Verification items for the finished model (mm, model axes). A direction names the side the tool comes from. Round coordinates to 2 decimals unless told otherwise and drop trailing zeros. Write each loop counter-clockwise with the first axis right and the second up, starting at its lowest first coordinate (ties: lowest second). Pieces come first, ordered by that corner, then holes. Notation, with made-up numbers: (-20.75, 0.5) - (13.25, 0.5) arc R8 cw to (13.25, 15.5) - close; hole circle Ø7 at (-33.5, -7). An arc over 180 degrees is marked (long way). Answer as a JSON object with one key per item and string values.
```python
from build123d import *

# Parameters (mm, degrees)
SKETCH1_R                = 13.6525
SKETCH1_R_2              = 10.668
BOSS_EXTRUDE1_DEPTH      = 63.5
SKETCH3_R                = 10.668
CUT_EXTRUDE2_DEPTH       = 69.85
BOSS_EXTRUDE2_REACH      = 81.247
BOSS_EXTRUDE2_END_RADIUS = 13.6525
SKETCH4_R                = 13.6525
SKETCH4_R_2              = 10.668
SKETCH5_W                = 1.905
SKETCH5_H                = 1.27
SKETCH6_W                = 1.27
SKETCH6_H                = 1.905
SKETCH7_W                = 1.27
SKETCH7_H                = 1.905


with BuildPart() as part:
    # Sketch1 → Boss-Extrude1 (new body)
    with BuildSketch(Plane(origin=(0, 0, 0), x_dir=(1, 0, 0), z_dir=(0, 1, 0))):
        with Locations(Location((0, 0, 0), (0, 0, 270))):
            Circle(SKETCH1_R)
        with Locations(Location((0, 0, 0), (0, 0, 270))):
            Circle(SKETCH1_R_2, mode=Mode.SUBTRACT)
    extrude(amount=BOSS_EXTRUDE1_DEPTH)

    # Sketch3 → Cut-Extrude2 (cut)
    with BuildSketch(Plane.XY):
        with Locations((0, 31.75)):
            Circle(SKETCH3_R)
    extrude(amount=-CUT_EXTRUDE2_DEPTH, mode=Mode.SUBTRACT)

    # Boss-Extrude2: up to this cylinder (the profile starts outside it)
    boss_extrude2_end = Plane(origin=(0, 31.75, 0), z_dir=(0, -1, 0)) * Cylinder(BOSS_EXTRUDE2_END_RADIUS, 190.799, mode=Mode.PRIVATE)
    # Sketch4 → Boss-Extrude2 (add, up to the surface)
    with BuildSketch(Plane.XY.offset(-31.75), mode=Mode.PRIVATE) as boss_extrude2_sk1:
        with Locations((0, 31.75)):
            Circle(SKETCH4_R)
        with Locations((0, 31.75)):
            Circle(SKETCH4_R_2, mode=Mode.SUBTRACT)
    boss_extrude2_tool1 = extrude(boss_extrude2_sk1.sketch, amount=BOSS_EXTRUDE2_REACH, mode=Mode.PRIVATE) - boss_extrude2_end
    add(boss_extrude2_tool1.solids().sort_by_distance((-13.266349, 31.75, -31.75))[0])

    # Sketch5 → Revolve1 (revolve)
    with BuildSketch(Plane(origin=(0, 0, 0), x_dir=(0, 0, -1), z_dir=(1, 0, 0)), mode=Mode.PRIVATE) as revolve1_sk:
        with Locations((11.7475, 21.717)):
            Rectangle(SKETCH5_W, SKETCH5_H)
    revolve(revolve1_sk.sketch.rotate(Axis((0, 31.75, -31.75), (0, 0, 1)), 90), axis=Axis((0, 31.75, -31.75), (0, 0, 1)))

    # Sketch6 → Revolve2 (revolve)
    with BuildSketch(Plane(origin=(0, 0, 0), x_dir=(0, 0, -1), z_dir=(1, 0, 0)), mode=Mode.PRIVATE) as revolve2_sk:
        with Locations((10.033, 43.4975)):
            Rectangle(SKETCH6_W, SKETCH6_H)
    revolve(revolve2_sk.sketch.rotate(Axis((0, 63.5, 0), (0, -1, 0)), 180), axis=Axis((0, 63.5, 0), (0, -1, 0)))

    # Sketch7 → Revolve3 (revolve)
    with BuildSketch(Plane(origin=(0, 0, 0), x_dir=(0, 0, -1), z_dir=(1, 0, 0)), mode=Mode.PRIVATE) as revolve3_sk:
        with Locations((-10.033, 20.0025)):
            Rectangle(SKETCH7_W, SKETCH7_H)
    revolve(revolve3_sk.sketch.rotate(Axis((0, 0, 0), (0, 1, 0)), 180), axis=Axis((0, 0, 0), (0, 1, 0)))

    # Sketch8 → Cut-Revolve1 (revolve, cut)
    with BuildSketch(Plane.XY, mode=Mode.PRIVATE) as cut_revolve1_sk:
        Polygon((13.6525, 0), (13.6525, 3.81), (12.7, 0), align=None)
    cut_revolve1 = revolve(cut_revolve1_sk.sketch.rotate(Axis((0, 0, 0), (0, 1, 0)), 90), axis=Axis((0, 0, 0), (0, 1, 0)), mode=Mode.SUBTRACT)

    # Mirror1: Cut-Revolve1 across plane
    add(cut_revolve1.mirror(Plane.ZX.offset(31.75)), mode=Mode.SUBTRACT)

    # Sketch9 → Cut-Revolve2 (revolve, cut)
    with BuildSketch(Plane(origin=(0, 0, 0), x_dir=(0, 0, -1), z_dir=(1, 0, 0)), mode=Mode.PRIVATE) as cut_revolve2_sk:
        Polygon((31.75, 18.0975), (27.94, 18.0975), (31.75, 19.05), align=None)
    revolve(cut_revolve2_sk.sketch.rotate(Axis((0, 31.75, -31.75), (0, 0, 1)), 270), axis=Axis((0, 31.75, -31.75), (0, 0, 1)), mode=Mode.SUBTRACT)


solid = part.part
```
Q1. Material ranges on line 1 along Y through (x, z) = (4.25, 9) (3 decimals); line 2 along Y through (x, z) = (0.5, -11.5); line 3 along X through (y, z) = (4, 0), recorded low to high. Write a range as [from, to].
Geometry check:
{"line 1": "y = [19.05, 20.955], [42.545, 44.45]", "line 2": "y = [0, 22.37], [41.13, 63.5]", "line 3": "x = [-13.65, -10.67], [10.67, 13.65]"}
Q2. Section check C-C, the plane x = 0. State how many separate pieces and enclosed holes the cut face has, then the cut area to 3 significant figures.
Geometry check:
{"separate pieces": "3", "enclosed holes": "0", "area": "427 mm2"}
Q3. Gauge pin test, flat ends, axial feed: P1, Ø1, axis at x = 3, y = 32.5, coming from the +Z side; P2, Ø1, axis at x = -7.5, y = 47.5, coming from the -Z side; P3, Ø1, axis at x = -1, z = -8.5, coming from the +Y side; P4, Ø5, axis at x = -10, y = 48, coming from the -Z side. Record the tip position at first contact, or that the pin passes through.
Geometry check:
{"P1": "stops at z = 13.42", "P2": "stops at z = -11.72", "P3": "passes through", "P4": "stops at z = -11.41"}
Q4. Release check for a two-part mould opening along Z. For faces 6 (the cylindrical face through (-6.491, 53.842, -8.466)), 7 (the flat face through (9, 20.955, -4)), 8 (the cylindrical face through (-2.313, 21.336, -22.358)), 9 (the cylindrical face through (4.101, 31.359, 13.022)) record: released by +Z, released by -Z, zero draft, split by the parting line, or undercut.
Geometry check:
{"face 6": "undercut", "face 7": "undercut", "face 8": "zero draft", "face 9": "split by the parting line"}
Q5. Set-up check for faces 1 (the flat face through (9, 0, -7)), 2 (the cylindrical face through (3.204, 31.599, 10.175)), 3 (the cylindrical face through (-6.491, 9.392, -8.466)), 4 (the cylindrical face through (-10.06, 40.98, -17.27)), 5 (the flat face through (9, 44.45, -4)): record each of +Z, -Z, +X, -X, +Y, -Y from which the full face is reachable in a straight line by a thin tool's end or side.
Geometry check:
{"face 1": "+Z, -Z, +X, -X, -Y", "face 2": "none", "face 3": "-Y", "face 4": "-Z", "face 5": "+Y"}
Q6. Section check D-D, the plane y = 14.5. Record the cut outline in (x, z) (1 decimal), then the cut area to 3 significant figures.
Geometry check:
{"outline": "circle Ø27.3 at (0, 0); hole circle Ø21.3 at (0, 0)", "area": "228 mm2"}
